```python
from build123d import *

# Parameters (mm, degrees)
BOSS_EXTRUDE1_DEPTH = 3.175
FILLET1_R           = 5
SKETCH3_W           = 3.629817958
SKETCH3_H           = 28
BOSS_EXTRUDE2_DEPTH = 20
SKETCH4_R           = 2.25
CUT_EXTRUDE1_DEPTH  = 3.629817958
FILLET2_R           = 3
FILLET3_R           = 2
SKETCH6_R           = 1.9
CUT_EXTRUDE2_DEPTH  = 3.175


with BuildPart() as part:
    # Sketch2 → Boss-Extrude1 (new body)
    with BuildSketch(Plane(origin=(0, 0, 0), x_dir=(0, 0, -1), z_dir=(1, 0, 0))):
        Polygon((-25.4, -95.305238918), (-6.35, -95.305238918), (-6.35, 0), (6.35, 0), (6.35, -108.005238918), (-25.4, -108.005238918), align=None)
    extrude(amount=-BOSS_EXTRUDE1_DEPTH)

    # Fillet1
    fillet1_edges = [part.edges().sort_by_distance(p)[0] for p in [
        (-1.5875, -95.305238918, 25.4),
        (-1.5875, -95.305238918, 6.35),
        (-1.5875, 0, -6.35),
    ]]
    fillet(fillet1_edges, radius=FILLET1_R)

    # Sketch3 → Boss-Extrude2 (add)
    with BuildSketch(Plane(origin=(0, 0, 0), x_dir=(0, 0, -1), z_dir=(1, 0, 0))):
        with Locations((-4.535091021, -14)):
            Rectangle(SKETCH3_W, SKETCH3_H)
    extrude(amount=BOSS_EXTRUDE2_DEPTH)

    # Sketch4 → Cut-Extrude1 (cut)
    with BuildSketch(Plane(origin=(0, 0, 2.720182042), x_dir=(-1, 0, 0), z_dir=(0, 0, -1))):
        with Locations((-15.75, -24)):
            Circle(SKETCH4_R)
        with Locations((-15.75, -4)):
            Circle(SKETCH4_R)
    extrude(amount=-CUT_EXTRUDE1_DEPTH, mode=Mode.SUBTRACT)

    # Fillet2
    fillet2_edges = [part.edges().sort_by_distance(p)[0] for p in [
        (0, -28, 4.535091021),
        (20, 0, 4.535091021),
        (20, -28, 4.535091021),
    ]]
    fillet(fillet2_edges, radius=FILLET2_R)

    # Fillet3
    fillet3_edges = [part.edges().sort_by_distance(p)[0] for p in [
        (-1.5875, -108.005238918, -6.35),
        (-1.5875, -108.005238918, 25.4),
    ]]
    fillet(fillet3_edges, radius=FILLET3_R)

    # Sketch6 → Cut-Extrude2 (cut)
    with BuildSketch(Plane(origin=(0, 0, 0), x_dir=(0, 0, -1), z_dir=(1, 0, 0))):
        with Locations((-5.405608289, -102.005238918)):
            Circle(SKETCH6_R)
        with Locations((-17.405608289, -102.005238918)):
            Circle(SKETCH6_R)
    extrude(amount=-CUT_EXTRUDE2_DEPTH, mode=Mode.SUBTRACT)


solid = part.part
```
Can you work these out from the model? Positions are in its coordinate system, mm. A direction names the side the tool comes from. Coordinates: 2 decimals unless noted, no trailing zeros. Loops run counter-clockwise (first coordinate to the right, second up) from the corner with the lowest first, then second, coordinate; pieces in that order, holes last.
Item 1: Please list where these lines run through material, in increasing order: L1, parallel to Y at x = 15.75, z = 4.05; L2, parallel to Y at x = 17, z = 5.5; L3, parallel to X at y = -100, z = 22.5 (3 decimals).
Answers below:
L1: y = -28 to -26.25, -21.75 to -6.25, -1.75 to 0
L2: y = -28 to -25.87, -22.13 to -5.87, -2.13 to 0
L3: x = -3.175 to 0
Item 2: Suppose I cut it at A-A (x = 15.75). Please give me the cut outline in (y, z).
Answers below:
outline: (-28, 2.72) - (-26.25, 2.72) - (-26.25, 6.35) - (-28, 6.35) - close; (-21.75, 2.72) - (-6.25, 2.72) - (-6.25, 6.35) - (-21.75, 6.35) - close; (-1.75, 2.72) - (0, 2.72) - (0, 6.35) - (-1.75, 6.35) - close
Item 3: Suppose I cut it at C-C (z = 18). Please give me the cut outline in (x, y) (3 decimals), then the cut area to 3 significant figures.
Answers below:
outline: (-3.175, -108.005) - (0, -108.005) - (0, -103.81) - (-3.175, -103.81) - close; (-3.175, -100.201) - (0, -100.201) - (0, -95.305) - (-3.175, -95.305) - close
area: 28.9 mm2
Item 4: Suppose I cut it at D-D (y = -12.5). Please give me the cut outline in (x, z) (3 decimals).
Answers below:
outline: (-3.175, -6.35) - (0, -6.35) - (0, 2.72) - (20, 2.72) - (20, 6.35) - (-3.175, 6.35) - close
Item 5: Suppose I cut it at B-B (y = -24). Please give me the cut outline in (x, z) (3 decimals).
Answers below:
outline: (-3.175, -6.35) - (0, -6.35) - (0, 2.72) - (13.5, 2.72) - (13.5, 6.35) - (-3.175, 6.35) - close; (18, 2.72) - (20, 2.72) - (20, 6.35) - (18, 6.35) - close
Item 6: Which directions (+Z, -Z, +X, -X, +Y, -Y) give clear straight access to the entire face, cutting with the end or side of a thin tool? Please do faces 1 (the face through (-1.57, -100.12, 17.65)), 2 (the face through (10, -28, 5)), 3 (the face through (6, -26, 6.35)), 4 (the face through (10, -12, 2.72)).
Answers below:
face 1: +X, -X
face 2: +Z, -Z, +X, -Y
face 3: +Z, +X, -X, +Y
face 4: -Z, +X, +Y, -Y
Item 7: If we mould it in two halves opening along X, with no side actions, what happens to faces 5 (the face through (-3.175, -53, 2)), 6 (the face through (0, -65, 2)), 7 (the face through (13.67, -4.86, 4.51))? For each: released by +X, released by -X, zero draft, split by the parting line, or undercut.
Answers below:
face 5: released by -X
face 6: released by +X
face 7: undercut
Item 8: I'm going to push flat-ended pins straight in: pin 1 (5 mm diameter, centred on x = 15.75, y = -4, fed in from +Z); pin 2 (9.5 mm diameter, centred on y = -33, z = 9, fed in from +X); pin 3 (8 mm diameter, centred on x = 1.5, y = -47, fed in from +Z). Where does each tip first touch, or does it pass through?
Answers below:
pin 1: stops at z = 6.35
pin 2: stops at x = 0.71
pin 3: stops at z = 6.35
